Input: part model. Units: mm. Frame: model coordinates. Face numbers are marked on the shaded views. A direction names the side the tool comes from. Round coordinates to 2 decimals unless told otherwise and drop trailing zeros. Loops run counter-clockwise (first coordinate to the right, second up) from the corner with the lowest first, then second, coordinate; pieces in that order, holes last. Notation, with made-up numbers: (13.25, 69.25) -> (35.25, 69.25) arc R15 ccw to (35.25, 78.25) -> close; hole circle Ø5 at (-5, -31.75). An arc over 180 degrees is marked (long way). Answer in a Markdown table with one row per item. Add a question column.
Q1. Section D-D, the plane x = -10. Output: boundary loops of the cut face in (y, z), and give its area (3 significant figures).
Q2. Pin query (flat end, axial travel): pin 1 (4 mm diameter, centred on x = 12.5, z = -1.5, fed in from -Y); pin 2 (3.5 mm diameter, centred on y = 8, z = 0.5, fed in from -X); pin 3 (2 mm diameter, centred on y = 0, z = -1, fed in from +X); pin 4 (2.5 mm diameter, centred on x = 0, y = 0, fed in from -Z). Return the tip coordinate at first contact, or that it passes through.
Q3. Ray query, L1, parallel to Y at x = 0, z = -1.75; L2, parallel to X at y = -8, z = -1.75; L3, parallel to Y at x = 7, z = -3. Return the intervals inside material, ascending. Write a range as from..to.
Q4. Mould query, pull axis Y, two halves, no side actions, for the marked faces 6, 7, 8 and 9. Classes: pulls with the +Y half, pulls with the -Y half, needs draft (parallel to the pull), parting line crosses it, or undercut.
Q5. Section C-C, the plane y = 4. Output: boundary loops of the cut face in (x, z), and give its area (3 significant figures).
Q6. Section B-B, the plane x = 0. Output: boundary loops of the cut face in (y, z).
Q7. Section A-A, the plane y = -8. Output: boundary loops of the cut face in (x, z), and give its area (3 significant figures).
Q8. Reachability of the marked faces 1, 2, 3, 4 and 5 from +Z, -Z, +X, -X, +Y, -Y: full face, straight path, thin tool, end or side. Return the list, or none.
Autodesk Inventor part; units mm, degrees
ref_plane "Work Plane1" through (0, -2, 0) normal (0, 1, 0) x (-1, 0, 0)
ref_plane "YZ Plane" through (0, 0, 0) normal (1, 0, 0) x (0, 1, 0)
ref_plane "XY Plane" through (0, 0, 0) normal (0, 0, 1) x (1, 0, 0)
sketch "Sketch1" plane through (0, 0, 0) normal (0, 0, 1) x (1, 0, 0)
  line L0 (-4, -12) -> (4, -12)
  line L1 (4, -12) -> (4, 12)
  line L2 (4, 12) -> (-4, 12)
  line L3 (-4, 12) -> (-4, -12)
  line L4 (-4, -12) -> (4, 12) construction
  line L5 (4, -12) -> (-4, 12) construction
  point P0 (0, 0)
  dimension "d0" = 8
  dimension "d1" = 24
extrude "Extrusion1" add sketch "Sketch1" along normal mid plane 8
ref_plane "Work Plane1" through (0, -2, 0) normal (0, 1, 0) x (-1, 0, 0)
sketch "Sketch3" plane through (0, -2, 0) normal (0, 1, 0) x (-1, 0, 0)
  line L0 (4, -4) -> (4, 4)
  line L1 (4, 4) -> (13, 4)
  arc A0 (13, -4) -> (13, 4) centre (13, 0) ccw
  line L2 (13, -4) -> (4, -4)
  line L3 (4, 4) -> (4, -4)
  line L4 (9, 0) -> (13, 0) construction
  line L5 (9, -2) -> (13, -2)
  line L6 (13, 2) -> (9, 2)
  arc A1 (9, 2) -> (9, -2) centre (9, 0) ccw
  arc A2 (13, -2) -> (13, 2) centre (13, 0) ccw
  point P0 (0, 0)
  point P1 (11, 0)
  dimension "d8" = 4
  dimension "d9" = 9
  dimension "d10" = 4
  dimension "d11" = 2
extrude "Extrusion2" add sketch "Sketch3" against normal blind 3
mirror "Mirror1" about plane through (0, 0, 0) normal (0, 1, 0) of "Extrusion2"
mirror "Mirror2" about plane through (0, 0, 0) normal (1, 0, 0) of "Extrusion2", "Mirror1"
sketch "Sketch4" plane through (0, 0, 4) normal (0, 0, 1) x (1, 0, 0)
  point P0 (0, 0)
  point P1 (0, -8)
  point P2 (0, 0)
  point P3 (0, 8)
  dimension "d14" = 8
  dimension "d15" = 8
hole "Hole1" at (0, -8, 4) at (0, 0, 4) at (0, 8, 4) direction (0, 0, -1) diameter 4 depth 8
sketch "Sketch5" plane through (4, -5, -4) normal (0, -1, 0) x (1, 0, 0)
  arc A0 (9, 2) -> (9, 6) centre (9, 4) ccw
  circle A1 centre (-14, 4) radius 2
  arc A2 (-13, 2) -> (-13, 6) centre (-13, 4) ccw
  arc A3 (-17, 6) -> (-17, 2) centre (-17, 4) ccw
  circle A4 centre (-14, 4) radius 2
  point P0 (-4, 4)
  point P1 (11, 4)
  point P2 (-11, 4)
  point P3 (-19, 4)
  dimension "d25" = 4
  dimension "d26" = 5
sketch "Sketch6" plane through (-13, 5, -4) normal (0, 1, 0) x (1, 0, 0)
  arc A0 (0, -2) -> (0, -6) centre (0, -4) ccw
  circle A1 centre (23, -4) radius 2
  arc A2 (26, -6) -> (26, -2) centre (26, -4) ccw
  arc A3 (22, -2) -> (22, -6) centre (22, -4) ccw
  point P0 (13, -4)
  point P1 (-2, -4)
  point P2 (28, -4)
  point P3 (20, -4)
  point P4 (28, -4)
  dimension "d28" = 4
  dimension "d31" = 5
properties part number "08"
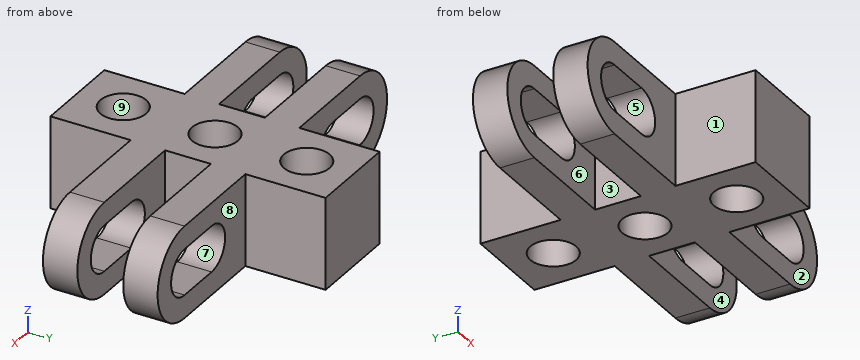
Answer block:
| question | item | result |
|---|---|---|
| 1 | outline | (-5, -4) -> (-2, -4) -> (-2, -2) -> (-5, -2) -> close; (-5, 2) -> (-2, 2) -> (-2, 4) -> (-5, 4) -> close; (2, -4) -> (5, -4) -> (5, -2) -> (2, -2) -> close; (2, 2) -> (5, 2) -> (5, 4) -> (2, 4) -> close |
| 1 | area | 24.0 mm^2 |
| 2 | pin 1 | y = -5 |
| 2 | pin 2 | x = -4 |
| 2 | pin 3 | x = 4 |
| 2 | pin 4 | through |
| 3 | L1 | -12..-10, -6..-2, 2..6, 10..12 |
| 3 | L2 | -4..-2, 2..4 |
| 3 | L3 | -5..-2, 2..5 |
| 4 | face 6 | undercut |
| 4 | face 7 | needs draft |
| 4 | face 8 | pulls with the +Y half |
| 4 | face 9 | undercut |
| 5 | outline | (-13, -4) -> (13, -4) arc R4 ccw to (13, 4) -> (-13, 4) arc R4 ccw to start; hole (-13, -2) -> (-9, -2) arc R2 ccw to (-9, 2) -> (-13, 2) arc R2 ccw to start; hole (9, -2) -> (13, -2) arc R2 ccw to (13, 2) -> (9, 2) arc R2 ccw to start |
| 5 | area | 201 mm^2 |
| 6 | outline | (-12, -4) -> (-10, -4) -> (-10, 4) -> (-12, 4) -> close; (-6, -4) -> (-2, -4) -> (-2, 4) -> (-6, 4) -> close; (2, -4) -> (6, -4) -> (6, 4) -> (2, 4) -> close; (10, -4) -> (12, -4) -> (12, 4) -> (10, 4) -> close |
| 7 | outline | (-4, -4) -> (-2, -4) -> (-2, 4) -> (-4, 4) -> close; (2, -4) -> (4, -4) -> (4, 4) -> (2, 4) -> close |
| 7 | area | 32.0 mm^2 |
| 8 | face 1 | +Z, -Z, -X, -Y |
| 8 | face 2 | +Z, -Z, +X, -Y |
| 8 | face 3 | +Z, -Z, -X |
| 8 | face 4 | +Z, -Z, +X |
| 8 | face 5 | +Y, -Y |
